Geometry check sheet. Reference: the model listing, model coordinates, mm. Face numbers are marked on the shaded views. Round coordinates to 2 decimals unless told otherwise and drop trailing zeros. Loops run counter-clockwise (first coordinate to the right, second up) from the corner with the lowest first, then second, coordinate; pieces in that order, holes last.
Autodesk Inventor part; units mm, degrees
ref_plane "Work Plane1" through (-17.5863, 0, 0) normal (0, -0.866, -0.5) x (1, 0, 0)
ref_plane "YZ Plane" through (0, 0, 0) normal (1, 0, 0) x (0, 1, 0)
ref_plane "XZ Plane" through (0, 0, 0) normal (0, 1, 0) x (-1, 0, 0)
sketch "Sketch1" plane through (0, 0, 0) normal (1, 0, 0) x (0, 1, 0)
  line L0 (-9.2376, 0) -> (-4.6188, 8)
  line L1 (-4.6188, 8) -> (4.6188, 8)
  line L2 (4.6188, 8) -> (9.2376, 0)
  line L3 (9.2376, 0) -> (4.6188, -8)
  line L4 (4.6188, -8) -> (-4.6188, -8)
  line L5 (-4.6188, -8) -> (-9.2376, 0)
  point P0 (0, 0)
  point P1 (0, 0)
  dimension "d0" = 18.4752
extrude "Body" add sketch "Sketch1" along normal blind 8.4
sketch "Sketch2" plane through (0, 0, 0) normal (0, 0, 1) x (1, 0, 0)
  line L0 (0, 4.6188) -> (0, 9.2376)
  line L1 (0, 9.2376) -> (8.4, 9.2376)
  line L2 (8.4, 4.6188) -> (8.4, 9.2376)
  line L3 (-1.68, 0) -> (10.08, 0)
  line L4 (1.1187, 9.2376) -> (0, 7.3)
  line L5 (7.2813, 9.2376) -> (8.4, 7.3)
  dimension "d3" = 30
  dimension "d4" = 30
  dimension "d5" = 14.6
  dimension "d6" = 14.6
revolve "Chamfer1" cut sketch "Sketch2" angle 360 about axis through (-10, 0, 0) along (1, 0, 0)
sketch "Sketch3" plane through (8.4, 0, 0) normal (1, 0, 0) x (0, 0, -1)
  arc A0 (-0.625, -1.0825) -> (0.625, -1.0825) centre (0, 0) ccw
hole "Thread" at (8.4, 0, 0) direction (-1, 0, 0) diameter 8.376 end through all
chamfer "Chamfer2" distance 0.8119 angle 30 1 edges at (8.4, 0, 4.188) measured on face at (8.4, 6.1818, -0.7506)
chamfer "Chamfer3" distance 0.8119 angle 30 1 edges at (0, 0, 4.188) measured on face at (0, 6.1818, -0.7506)
ref_plane "Work Plane1" through (-17.5863, 0, 0) normal (0, -0.866, -0.5) x (1, 0, 0)
equation "\"d0\" = 1.1547 * SW"
equation "\"d1\" = KOH"
equation "\"d3\" = ANG1"
equation "\"d4\" = ANG2"
equation "\"d5\" = SW0"
equation "\"d6\" = SW01"
equation "\"d8\" = -0.5 * GD1 + 0.5 * NND"
equation "\"d40\" = -0.5 * GD1 + 0.5 * NND"
equation "\"d10\" = -0.5 * GD1 + 0.5 * NND"
equation "\"d41\" = -0.5 * GD1 + 0.5 * NND"
equation "\"ANG1\" = 30deg"
equation "\"ANG2\" = 30deg"
equation "\"KOH\" = 8.4"
equation "\"SW\" = 16"
equation "\"SW0\" = 14.6"
equation "\"SW01\" = 14.6"
equation "\"GUL\" = 0.541266 * PTC"
equation "\"TOA\" = 30deg"
equation "\"PTC\" = 1.5"
equation "\"E0\" = 1.155 * SW"
equation "\"GAL\" = 0.541266 * PTC"
properties part number "ISO 4032 - M10" material "Stainless Steel, 440C"
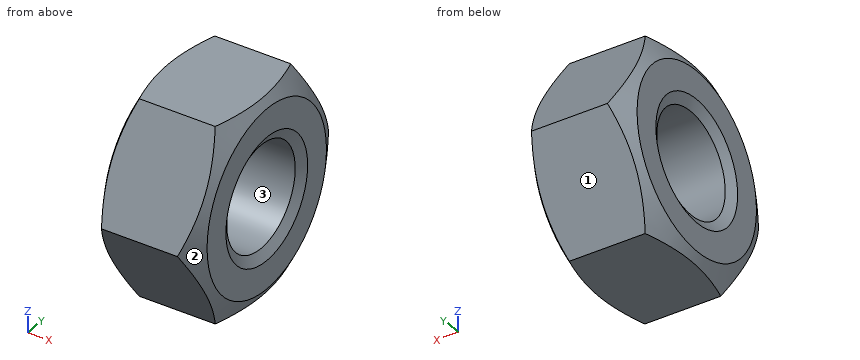
1) Sectioned sample at A-A, the plane y = 0. Record the cut outline in (x, z).
Report:
outline: (0, -7.3) - (0.4, -8) - (8, -8) - (8.4, -7.3) - (8.4, -5) - (7.93, -4.19) - (0.47, -4.19) - (0, -5) - close; (0, 5) - (0.47, 4.19) - (7.93, 4.19) - (8.4, 5) - (8.4, 7.3) - (8, 8) - (0.4, 8) - (0, 7.3) - close
2) Gauge pin test, flat ends, axial feed: pin 1 (4 mm diameter, centred on x = 4.5, z = 6.5, fed in from -Y); pin 2 (1 mm diameter, centred on x = 2.5, z = 6.5, fed in from +Y); pin 3 (1 mm diameter, centred on x = 3, z = 2.5, fed in from +Y). Record the tip position at first contact, or that the pin passes through.
Report:
pin 1: stops at y = -6.64
pin 2: stops at y = 5.77
pin 3: stops at y = 8.08
3) Sectioned sample at B-B, the plane x = 2.75. Record the cut outline in (y, z).
Report:
outline: (-9.24, 0) - (-4.62, -8) - (4.62, -8) - (9.24, 0) - (4.62, 8) - (-4.62, 8) - close; hole circle Ø8.38 at (0, 0)
4) Scan lines: line 1 along Z through (x, y) = (4.5, 0); line 2 along Y through (x, z) = (3, -1.25); line 3 along Y through (x, z) = (2, -3.75). Record each from-to range of solid material in increasing order.
Report:
line 1: z = -8 to -4.19, 4.19 to 8
line 2: y = -8.52 to -4, 4 to 8.52
line 3: y = -7.07 to -1.86, 1.86 to 7.07
5) Mould release check, pull along Z, two halves, no side actions. Record for the marked faces 1, 2 and 3: +Z half, -Z half, draft (parallel to the pull), parting line (faces both ways), or undercut.
Report:
face 1: -Z half
face 2: parting line
face 3: undercut
